Source: CAD feature listing. Evaluate the final solid. Frame: model axes, mm. A direction names the side the tool comes from. Coordinates: 2 decimals unless noted, no trailing zeros. Loops run counter-clockwise (first coordinate to the right, second up) from the corner with the lowest first, then second, coordinate; pieces in that order, holes last. Notation, with made-up numbers: M -25,-9 L -2,-9 A9 ccw -2,2 Z; hole C -14,71.25 d1. An arc over 180 degrees is marked long. One line per question, with ' | ' between items. Start each with the question number.
1. Section query C-C, the plane y = -2.5. Output: boundary loops of the cut face in (x, z).
2. Section query A-A, the plane y = 11. Output: boundary loops of the cut face in (x, z).
3. Pin query (flat end, axial travel): P1, Ø4, axis at x = 29, z = -5, coming from the +Y side; P2, Ø6, axis at x = 43, z = -13.5, coming from the -Y side; P3, Ø1.5, axis at y = 7.5, z = -25.5, coming from the -X side; P4, Ø6, axis at x = -11.5, z = -13.5, coming from the +Y side. Return the tip coordinate at first contact, or that it passes through.
4. Ray query, probe 1 along X at (y, z) = (10.25, -23); probe 2 along Z at (x, y) = (20, 1.5); probe 3 along Z at (x, y) = (13.5, 1). Return the intervals inside material, ascending.
5. Section query B-B, the plane z = -24.5. Output: boundary loops of the cut face in (x, y).
6. Mould query, pull axis X, two halves, no side actions, for faces 5 (the cylindrical face through (29.79, -1.078, -33.127)), 6 (the flat face through (75, 2, 0)), 7 (the flat face through (0, 2, -10)), 8 (the flat face through (-15, 3.8, -15.8)). Classes: pulls with the +X half, pulls with the -X half, needs draft (parallel to the pull), parting line crosses it, or undercut.
7. Section query D-D, the plane x = -42. Output: boundary loops of the cut face in (y, z).
8. Access query for faces 1 (the flat face through (-60, 2, -10)), 2 (the cylindrical face through (29.79, 2.774, -27.027)), 3 (the flat face through (60, 2, -10)), 4 (the flat face through (-1, 5, 0)). Directions: +Z, -Z, +X, -X, +Y, -Y. A direction counts if a zero-diameter tool reaches every point of the face in a straight line with its end or side. Return the directions, or none.
```python
from build123d import *

# Parameters (mm, degrees)
SKETCH1_W           = 150
SKETCH1_H           = 20
BOSS_EXTRUDE1_DEPTH = 5
BOSS_EXTRUDE2_START = -60
SKETCH2_R           = 12
SKETCH2_R_2         = 6
BOSS_EXTRUDE2_DEPTH = 30
LPATTERN1_COUNT     = 2
LPATTERN1_PITCH     = 60


with BuildPart() as part:
    # Sketch1 → Boss-Extrude1 (new body)
    with BuildSketch(Plane(origin=(0, 0, 0), x_dir=(1, 0, 0), z_dir=(0, 1, 0))):
        Rectangle(SKETCH1_W, SKETCH1_H)
    extrude(amount=BOSS_EXTRUDE1_DEPTH)

    # Sketch2 → Boss-Extrude2 (add)
    with BuildSketch(Plane(origin=(75, 0, 0), x_dir=(0, 0, -1), z_dir=(1, 0, 0)).offset(BOSS_EXTRUDE2_START)):
        with Locations((21.303604064, 0.97153439)):
            Circle(SKETCH2_R)
        with Locations((21.303604064, 0.97153439)):
            Circle(SKETCH2_R_2, mode=Mode.SUBTRACT)
    boss_extrude2 = extrude(amount=BOSS_EXTRUDE2_DEPTH)

    # LPattern1: Boss-Extrude2 ×2
    with Locations(*[(-i * LPATTERN1_PITCH, 0, 0) for i in range(1, LPATTERN1_COUNT)]):
        add(boss_extrude2)


solid = part.part
```
Taken from the geometry:
1) outline: M -45,-32.79 L -15,-32.79 L -15,-26.2 L -45,-26.2 Z; M -45,-16.41 L -15,-16.41 L -15,-9.82 L -45,-9.82 Z; M 15,-32.79 L 45,-32.79 L 45,-26.2 L 15,-26.2 Z; M 15,-16.41 L 45,-16.41 L 45,-9.82 L 15,-9.82 Z
2) outline: M -45,-27.89 L -15,-27.89 L -15,-14.71 L -45,-14.71 Z; M 15,-27.89 L 45,-27.89 L 45,-14.71 L 15,-14.71 Z
3) P1: y = 5 | P2: y = -10.03 | P3: x = -45 | P4: through
4) probe 1: -45 to -15, 15 to 45 | probe 2: -33.29 to -27.28, -15.33 to 10 | probe 3: -10 to 10
5) outline: M -45,-10.59 L -15,-10.59 L -15,-4.11 L -45,-4.11 Z; M -45,6.05 L -15,6.05 L -15,12.54 L -45,12.54 Z; M 15,-10.59 L 45,-10.59 L 45,-4.11 L 15,-4.11 Z; M 15,6.05 L 45,6.05 L 45,12.54 L 15,12.54 Z
6) face 5: needs draft | face 6: pulls with the +X half | face 7: undercut | face 8: undercut
7) outline: M 0,-9.34 A12 ccw long 5,-10 L 5,10 L 0,10 Z; hole C 0.97,-21.3 d12
8) face 1: -Z, -X, +Y, -Y | face 2: +X, -X | face 3: -Z, +X, +Y, -Y | face 4: +Z, +X, -X, +Y
